Could you check a few things on this model? Use its own coordinates, in mm. Face numbers are marked on the shaded views. A direction names the side the tool comes from. Round coordinates to 2 decimals unless told otherwise and drop trailing zeros. Order: outer loops, then holes, each group sorted by start corner. A loop starts at its lowest first (then second) coordinate and runs counter-clockwise, first axis right, second up. Notation, with made-up numbers: (24, 27.5) -> (64, 27.5) arc R32 cw to (64, 55.5) -> close; hole circle Ø2 at (-20.75, 20). An arc over 180 degrees is marked (long way). One line per question, with ' | ' between items.
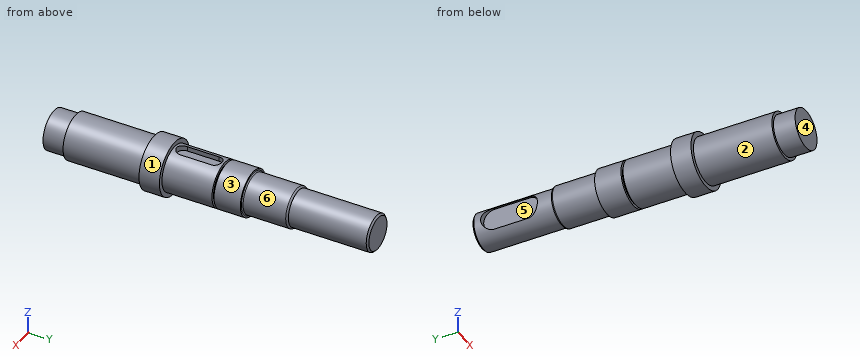
```python
from build123d import *

# Parameters (mm, degrees)
CHAMFER1_SIZE      = 1.5
FILLET2_R          = 1.5
CUT_EXTRUDE1_DEPTH = 5
CUT_EXTRUDE2_DEPTH = 5
FILLET4_R          = 1


with BuildPart() as part:
    # Sketch1 → Revolve1 (revolve)
    with BuildSketch(Plane.XY):
        Polygon((0, 0), (17.5, 0), (17.5, 19), (20, 19), (20, 88), (24, 88), (24, 106), (20, 106), (20, 150), (17.5, 150), (17.5, 151.8), (20, 151.8), (20, 175), (17.5, 175), (17.5, 215), (16, 215), (16, 285), (0, 285), align=None)
    revolve(axis=Axis((0, 0, 0), (0, 1, 0)))

    # Chamfer1
    chamfer1_edges = [part.edges().sort_by_distance(p)[0] for p in [
        (-16, 285, 0),
    ]]
    chamfer(chamfer1_edges, length=CHAMFER1_SIZE)

    # Fillet2
    fillet2_edges = [part.edges().sort_by_distance(p)[0] for p in [
        (-17.5, 215, 0),
    ]]
    fillet(fillet2_edges, radius=FILLET2_R - 0.0001)  # a hair under: the kernel refuses the full size

    # Sketch3 → Cut-Extrude1 (cut)
    with BuildSketch(Plane.XY.offset(20)):
        with BuildLine():
            Line((6, 142), (6, 114))
            ThreePointArc((6, 114), (0, 108), (-6, 114))
            Line((-6, 114), (-6, 142))
            ThreePointArc((-6, 142), (0, 148), (6, 142))
        make_face()
    extrude(amount=-CUT_EXTRUDE1_DEPTH, mode=Mode.SUBTRACT)

    # Sketch4 → Cut-Extrude2 (cut)
    with BuildSketch(Plane(origin=(-16, 0, 0), x_dir=(0, 0, -1), z_dir=(1, 0, 0))):
        with BuildLine():
            Line((10, 267.5), (10, 237.5))
            ThreePointArc((10, 237.5), (0, 227.5), (-10, 237.5))
            Line((-10, 237.5), (-10, 267.5))
            ThreePointArc((-10, 267.5), (0, 277.5), (10, 267.5))
        make_face()
    extrude(amount=CUT_EXTRUDE2_DEPTH, mode=Mode.SUBTRACT)

    # Fillet4
    fillet4_edges = [part.edges().sort_by_distance(p)[0] for p in [
        (-17.5, 175, 0),
    ]]
    fillet(fillet4_edges, radius=FILLET4_R)


solid = part.part
```
1. I want a section at D-D on y = 233. List the corners of the cut face in (x, z) for me.
From the geometry:
outline: (-13.28, -8.93) arc R16 ccw (long way) to (-13.28, 8.93) -> (-11, 8.93) -> (-11, -8.93) -> close
2. I want a section at B-B on y = 186. List the corners of the cut face in (x, z) for me.
From the geometry:
outline: circle Ø35 at (0, 0)
3. On a 3-axis mill with a long thin cutter (end or side, diameter ignored), from which of +Z, -Z, +X, -X, +Y, -Y can I reach the whole of each face in a straight line? I mean the marked faces 1, 2 and 3. Say none if no direction works.
From the geometry:
face 1: +Y, -Y | face 2: -Y | face 3: +Y
4. I need wall thicknesses on probe 1 along Y at (x, z) = (-17.5, 9); probe 2 along X at (y, z) = (135.5, -0.5); probe 3 along Y at (x, z) = (-19, -8). Which ranges of each line are inside material? Lowest first, please.
From the geometry:
probe 1: y = 19 to 150, 151.8 to 175 | probe 2: x = -19.99 to 19.99 | probe 3: y = 88 to 106
5. I'm going to push flat-ended pins straight in: pin 1 (2 mm diameter, centred on y = 125.5, z = 18, fed in from +X); pin 2 (1.6 mm diameter, centred on x = -12, y = 245.5, fed in from -Z); pin 3 (1 mm diameter, centred on x = -0.5, y = 243.5, fed in from -Z). Where does each tip first touch, or does it pass through?
From the geometry:
pin 1: stops at x = 10.54 | pin 2: stops at z = -11.43 | pin 3: stops at z = -16
6. I want a section at A-A on y = 136. List the corners of the cut face in (x, z) for me, and give its area (3 significant figures).
From the geometry:
outline: (-6, 15) -> (-6, 19.08) arc R20 ccw (long way) to (6, 19.08) -> (6, 15) -> close | area: 1,200 mm²
7. If we mould it in two halves opening along Z, with no side actions, what happens to the marked faces 4, 5 and 6? For each: pulls with the +Z half, pulls with the -Z half, needs draft (parallel to the pull), parting line crosses it, or undercut.
From the geometry:
face 4: needs draft | face 5: undercut | face 6: parting line crosses it
8. I want a section at C-C on y = 55.5. List the corners of the cut face in (x, z) for me.
From the geometry:
outline: circle Ø40 at (0, 0)
